Geometry check sheet. Reference: drawing and pictorial views, mm from the part's lowest x, y, z. Give positions to 0.01 mm unless a question says otherwise; leave off trailing zeros. Loops run counter-clockwise (first coordinate to the right, second up) from the corner with the lowest first, then second, coordinate; pieces in that order, holes last. Notation, with made-up numbers: (63.25, -16) - (75.25, -16) arc R24 cw to (75.25, 20) - close; hole circle Ø11 at (64.5, 48). An arc over 180 degrees is marked (long way). One line per question, with ' | ' between items. Start each with the question number.
1. Section check A-A, the plane x = 0.55. Enter the section's corners in (y, z) (1 decimal), then the cut area to 3 significant figures.
2. Thickness scan on line 1 along Z through (x, y) = (1.55, 3); line 2 along Y through (x, z) = (2.75, 2.25) (1 decimal); line 3 along Z through (x, y) = (1.05, 4.75). Record the ranges inside material, lowest first. Write a range as from..to.
3. Section check C-C, the plane x = 2.7. Enter the section's corners in (y, z) (1 decimal).
4. Mould release check, pull along Y, two halves, no side actions. Record for the marked faces 1, 2 and 3: +Y half, -Y half, draft (parallel to the pull), parting line (faces both ways), or undercut.
5. Section check B-B, the plane x = 2.2. Enter the section's corners in (y, z).
6. Depth check by flat-ended pin: pin 1 Ø1.5 at (x, y) = (2.5, 7.5) entering from -Z; pin 2 Ø2.5 at (y, z) = (4.04, 3.5) entering from -X; pin 3 Ø1.5 at (x, y) = (1, 6.5) entering from -Z. Enter the tip coordinate at first touch or a pass-through.
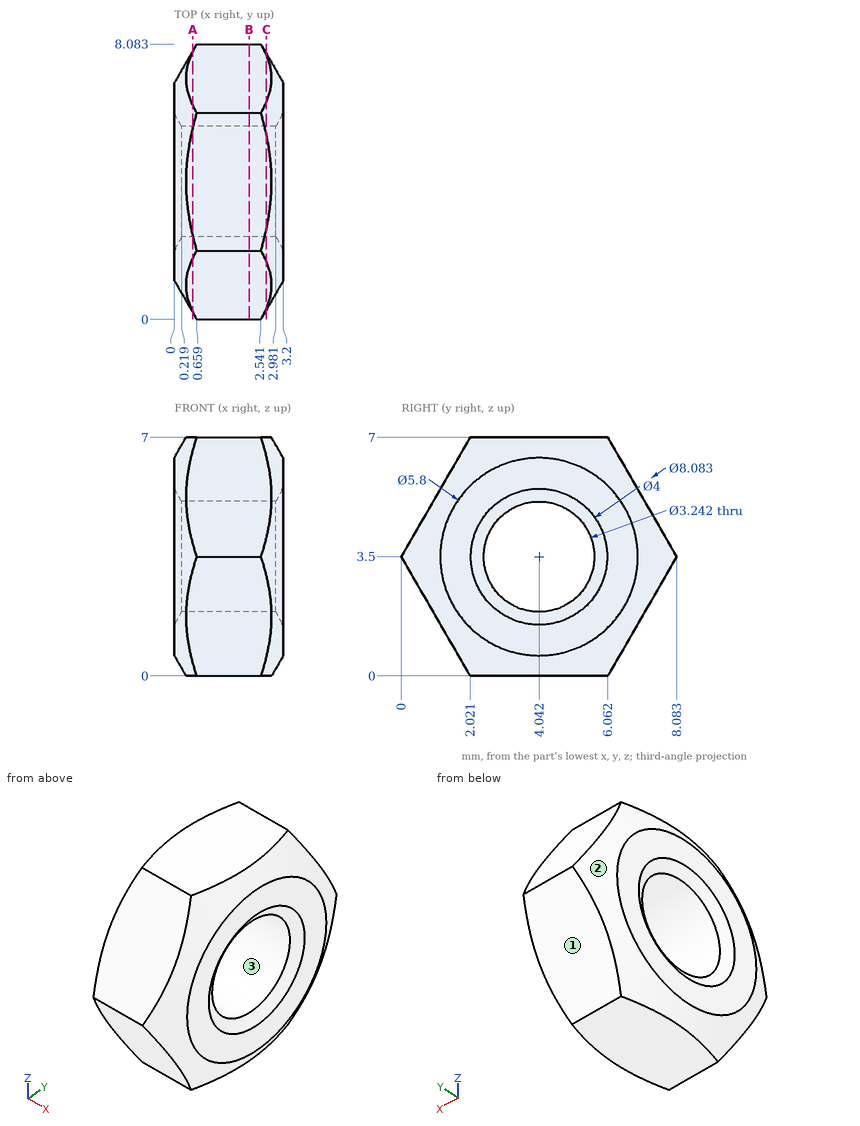
Results list:
1) outline: (0.2, 3.1) - (1.8, 0.4) arc R3.9 ccw to (2.4, 0) - (5.7, 0) arc R3.9 ccw to (6.3, 0.4) - (7.9, 3.1) arc R3.9 ccw to (7.9, 3.9) - (6.3, 6.6) arc R3.9 ccw to (5.7, 7) - (2.4, 7) arc R3.9 ccw to (1.8, 6.6) - (0.2, 3.9) arc R3.9 ccw to start; hole circle Ø3.2 at (4, 3.5) | area: 33.8 mm²
2) line 1: 0..2.26, 4.74..7 | line 2: 0.7..3, 5.1..7.4 | line 3: 0..2.04, 4.96..7
3) outline: (0.3, 3) - (1.7, 0.5) arc R3.8 ccw to (2.7, 0) - (5.4, 0) arc R3.8 ccw to (6.4, 0.5) - (7.8, 3) arc R3.8 ccw to (7.8, 4) - (6.4, 6.5) arc R3.8 ccw to (5.4, 7) - (2.7, 7) arc R3.8 ccw to (1.7, 6.5) - (0.3, 4) arc R3.8 ccw to start; hole circle Ø3.2 at (4, 3.5)
4) face 1: +Y half | face 2: parting line | face 3: undercut
5) outline: (0, 3.5) - (2.02, 0) - (6.06, 0) - (8.08, 3.5) - (6.06, 7) - (2.02, 7) - close; hole circle Ø3.24 at (4.04, 3.5)
6) pin 1: z = 1.19 | pin 2: through | pin 3: z = 0
